Could you check a few things on this model? Use its own coordinates, in mm. A direction names the side the tool comes from. Coordinates: 2 decimals unless noted, no trailing zeros. Loops run counter-clockwise (first coordinate to the right, second up) from the corner with the lowest first, then second, coordinate; pieces in that order, holes last. Notation, with made-up numbers: (17.5, -13.75) - (29.5, -13.75) arc R22 ccw to (29.5, 19.25) - close; hole circle Ø6 at (-24.75, 0). An arc over 180 degrees is marked (long way). One line per question, with ' | ' between items. Start each with the question number.
1. I want a section at B-B, the plane y = -21. Write out the boundary of the cut face in (x, z).
2. I'm going to push flat-ended pins straight in: P1, Ø2, axis at y = -10, z = 5, coming from the +X side; P2, Ø3, axis at x = -10.5, y = -10, coming from the +Z side; P3, Ø7, axis at x = 9.5, y = -7.5, coming from the +Z side. Where does each tip first touch, or does it pass through?
3. Which directions (+Z, -Z, +X, -X, +Y, -Y) give clear straight access to the entire face, cutting with the end or side of a thin tool? Please do faces 1 (the flat face through (-9, -12, 2.476)), 2 (the flat face through (0.254, -12, 7)), 3 (the flat face through (6.35, -12, 6)).
4. Please list where these lines run through material, in increasing order: L1, parallel to X at y = -12.25, z = 8.25; L2, parallel to Z at x = 11.75, y = -2.25; L3, parallel to X at y = -21.5, z = 9.75. Write a range as [from, to].
5. I want a section at C-C, the plane x = 10.25. Write out the boundary of the cut face in (y, z).
6. We'd pull the mould along X, two halves only. Please class faces 4 (the flat face through (2, -12, 11.262)), 5 (the flat face through (-0.254, -12, 7)), 6 (the flat face through (-12.7, -12, 1)): pulls with the +X half, pulls with the -X half, needs draft (parallel to the pull), parting line crosses it, or undercut.
7. I want a section at D-D, the plane z = 10.75. Write out the boundary of the cut face in (x, y), then the cut area to 3 significant figures.
8. I want a section at A-A, the plane z = 4. Write out the boundary of the cut face in (x, y), then the cut area to 3 significant figures.
from build123d import *

# Parameters (mm, degrees)
F0_W     = 12.7
F0_H     = 8.786774
F1_DEPTH = 24.13
F2_W     = 0.508
F2_H     = 24.13
F3_DEPTH = 8.89
F4_SIZE  = 2.54


with BuildPart() as f1:
    # F0 (on Front) → F1 (new body)
    with BuildSketch(Plane.XZ):
        Polygon((-12.7, 2.475597), (-12.7, -0.445403), (12.7, -0.445403), (12.7, 2.475597), (6.35, 2.475597), (-6.35, 2.475597), align=None)
        with Locations((0, 6.868984)):
            Rectangle(F0_W, F0_H)
    extrude(amount=F1_DEPTH)

    # F2 (on face) → F3 (cut)
    with BuildSketch(Plane.XY.offset(11.262371)):
        with Locations((0, -12.065)):
            Rectangle(F2_W, F2_H)
    extrude(amount=-F3_DEPTH, mode=Mode.SUBTRACT)

    # F4
    f4_edges = [f1.edges().sort_by_distance(p)[0] for p in [
        (-6.35, -12.065, 11.262371),
        (6.35, -12.065, 11.262371),
    ]]
    chamfer(f4_edges, length=F4_SIZE)


solid = f1.part
Results are:
1) outline: (-12.7, -0.45) - (12.7, -0.45) - (12.7, 2.48) - (6.35, 2.48) - (6.35, 8.72) - (3.81, 11.26) - (0.25, 11.26) - (0.25, 2.37) - (-0.25, 2.37) - (-0.25, 11.26) - (-3.81, 11.26) - (-6.35, 8.72) - (-6.35, 2.48) - (-12.7, 2.48) - close
2) P1: stops at x = 6.35 | P2: stops at z = 2.48 | P3: stops at z = 9.07
3) face 1: +Z, -X, +Y, -Y | face 2: +Z, +Y, -Y | face 3: +Z, +X, +Y, -Y
4) L1: x = [-6.35, -0.25], [0.25, 6.35] | L2: z = [-0.45, 2.48] | L3: x = [-5.32, -0.25], [0.25, 5.32]
5) outline: (-24.13, -0.45) - (0, -0.45) - (0, 2.48) - (-24.13, 2.48) - close
6) face 4: needs draft | face 5: undercut | face 6: pulls with the -X half
7) outline: (-4.32, -24.13) - (-0.25, -24.13) - (-0.25, 0) - (-4.32, 0) - close; (0.25, -24.13) - (4.32, -24.13) - (4.32, 0) - (0.25, 0) - close | area: 196 mm2
8) outline: (-6.35, -24.13) - (-0.25, -24.13) - (-0.25, 0) - (-6.35, 0) - close; (0.25, -24.13) - (6.35, -24.13) - (6.35, 0) - (0.25, 0) - close | area: 294 mm2
